Verification items for the finished model (mm, model axes). A direction names the side the tool comes from. Round coordinates to 2 decimals unless told otherwise and drop trailing zeros. Order: outer loops, then holes, each group sorted by start corner. A loop starts at its lowest first (then second) coordinate and runs counter-clockwise, first axis right, second up. Notation, with made-up numbers: (8.5, 50.5) -> (61.5, 50.5) arc R26 ccw to (61.5, 82.5) -> close; hole circle Ø4 at (-29.75, -3). An arc over 180 degrees is marked (long way). Put each result on its own line as item: value.
from build123d import *

# Parameters (mm, degrees)
SKETCH004_W     = 15.5
SKETCH004_H     = 10.4
PAD003_DEPTH    = 19.5
SKETCH005_W     = 10.4
SKETCH005_H     = 15.5
POCKET_DEPTH    = 45
SKETCH006_W     = 10.4
SKETCH006_H     = 15.5
POCKET001_DEPTH = 45


with BuildPart() as part:
    # Sketch004 → Pad003 (new body)
    with BuildSketch(Plane.XY):
        Polygon((-9.75, 7.2), (-9.75, -47.2), (4.65, -47.2), (4.65, -7.2), (49.75, -7.2), (49.75, 7.2), align=None)
        Rectangle(SKETCH004_W, SKETCH004_H, mode=Mode.SUBTRACT)
    extrude(amount=PAD003_DEPTH)

    # Sketch005 (on Face2 of Pad003) → Pocket (cut)
    with BuildSketch(Plane.XZ.offset(47.2)):
        with Locations((-2.55, 9.75)):
            Rectangle(SKETCH005_W, SKETCH005_H)
    extrude(amount=-POCKET_DEPTH, mode=Mode.SUBTRACT)

    # Sketch006 (on Face6 of Pocket) → Pocket001 (cut)
    with BuildSketch(Plane.YZ.offset(49.75)):
        with Locations((0, 9.75)):
            Rectangle(SKETCH006_W, SKETCH006_H)
    extrude(amount=-POCKET001_DEPTH, mode=Mode.SUBTRACT)


solid = part.part
Item 1: Section check B-B on z = 10.5. Record the boundary of the cut face in (x, y), then the cut area to 3 significant figures.
Check sheet entries:
outline: (-9.75, -47.2) -> (-7.75, -47.2) -> (-7.75, 5.2) -> (49.75, 5.2) -> (49.75, 7.2) -> (-9.75, 7.2) -> close; (2.65, -47.2) -> (4.65, -47.2) -> (4.65, -7.2) -> (49.75, -7.2) -> (49.75, -5.2) -> (2.65, -5.2) -> close
area: 398 mm^2
Item 2: Gauge pin test, flat ends, axial feed: pin 1 Ø10 at (x, z) = (21.5, 5) entering from -Y; pin 2 Ø4 at (y, z) = (-11, 15.5) entering from +X. Record the tip position at first contact, or that the pin passes through.
Check sheet entries:
pin 1: stops at y = -7.2
pin 2: stops at x = 4.65
Item 3: Tool access check on faces 1 (the flat face through (-3, -26, 2)), 2 (the flat face through (29, 0, 17.5)), 3 (the flat face through (27, -7.2, 10)), 4 (the flat face through (7.75, 0, 1)). Record the directions out of +Z, -Z, +X, -X, +Y, -Y that give a thin tool (end or side, any length) a straight path to the whole face; none if there is none.
Check sheet entries:
face 1: -Y
face 2: +X
face 3: +Z, -Z, +X, -Y
face 4: +Z, -Z
Item 4: Section check D-D on x = 35. Record the boundary of the cut face in (y, z), then the cut area to 3 significant figures.
Check sheet entries:
outline: (-7.2, 0) -> (7.2, 0) -> (7.2, 19.5) -> (-7.2, 19.5) -> close; hole (-5.2, 2) -> (5.2, 2) -> (5.2, 17.5) -> (-5.2, 17.5) -> close
area: 120 mm^2
Item 5: Section check A-A on x = 3.5. Record the boundary of the cut face in (y, z), then the cut area to 3 significant figures.
Check sheet entries:
outline: (-47.2, 0) -> (-5.2, 0) -> (-5.2, 19.5) -> (-47.2, 19.5) -> close; (5.2, 0) -> (7.2, 0) -> (7.2, 19.5) -> (5.2, 19.5) -> close
area: 858 mm^2
Item 6: Material ranges on L1, parallel to Z at x = 0, y = -40.5; L2, parallel to Y at x = 22.5, z = 7.5; L3, parallel to X at y = -45, z = 14.5, recorded low to high. Write a range as [from, to].
Check sheet entries:
L1: z = [0, 2], [17.5, 19.5]
L2: y = [-7.2, -5.2], [5.2, 7.2]
L3: x = [-9.75, -7.75], [2.65, 4.65]
Item 7: Section check C-C on y = -23.5. Record the boundary of the cut face in (x, z), then the cut area to 3 significant figures.
Check sheet entries:
outline: (-9.75, 0) -> (4.65, 0) -> (4.65, 19.5) -> (-9.75, 19.5) -> close; hole (-7.75, 2) -> (2.65, 2) -> (2.65, 17.5) -> (-7.75, 17.5) -> close
area: 120 mm^2
Item 8: Release check for a two-part mould opening along X. For faces 5 (the flat face through (-7.75, -21, 10)), 6 (the flat face through (49.75, 6, 10)), 7 (the flat face through (-9.75, -20, 10)), 8 (the flat face through (29, 0, 2)) record: +X half, -X half, draft (parallel to the pull), parting line (faces both ways), or undercut.
Check sheet entries:
face 5: undercut
face 6: +X half
face 7: -X half
face 8: draft
